```python
from build123d import *

# Parameters (mm, degrees)
F0_R      = 30
F1_DEPTH  = 5
F3_DEPTH  = 95
F4_R      = 25
F5_DEPTH  = 5
F6_R      = 37.5
F6_R_2    = 25
F7_DEPTH  = 10
F8_R      = 25
F9_DEPTH  = 30
F10_R     = 37.5
F11_DEPTH = 10
F12_R     = 25
F13_DEPTH = 5
F15_DEPTH = 95
F16_R     = 30
F17_DEPTH = 5
F18_R     = 20
F19_DEPTH = 30
F20_R     = 20
F21_DEPTH = 30
F22_R     = 10


with BuildPart() as f1:
    # F0 (on Right) → F1 (new body)
    with BuildSketch(Plane.YZ):
        Circle(F0_R)
    extrude(amount=F1_DEPTH)

    # F2 (on face) → F3 (join)
    with BuildSketch(Plane.YZ.offset(5)):
        with BuildLine():
            ThreePointArc((60.0712170477, -35.9367344428), (67.4721616422, -18.6415504541), (70, 0))
            ThreePointArc((70, 0), (37.1422350498, 59.333417022), (-30.5844107288, 62.9650206096))
            Line((-30.5844107288, 62.9650206096), (60.0712170477, -35.9367344428))
        make_face()
        with BuildLine():
            Line((60.0712170477, -35.9367344428), (-30.5844107288, 62.9650206096))
            ThreePointArc((-30.5844107288, 62.9650206096), (-47.2995007919, 51.601911058), (-60.0712170477, 35.9367344428))
            Line((-60.0712170477, 35.9367344428), (30.5844107288, -62.9650206096))
            ThreePointArc((30.5844107288, -62.9650206096), (47.2995007919, -51.601911058), (60.0712170477, -35.9367344428))
        make_face()
        with BuildLine():
            ThreePointArc((-60.0712170477, 35.9367344428), (-47.2995007919, 51.601911058), (-30.5844107288, 62.9650206096))
            Line((-30.5844107288, 62.9650206096), (-39.3131691742, 72.4877557211))
            Line((-39.3131691742, 72.4877557211), (-68.7999754931, 45.4594695543))
            Line((-68.7999754931, 45.4594695543), (-60.0712170477, 35.9367344428))
        make_face()
        with BuildLine():
            Line((68.7999754931, -45.4594695543), (60.0712170477, -35.9367344428))
            ThreePointArc((60.0712170477, -35.9367344428), (47.2995007919, -51.601911058), (30.5844107288, -62.9650206096))
            Line((30.5844107288, -62.9650206096), (39.3131691742, -72.4877557211))
            Line((39.3131691742, -72.4877557211), (68.7999754931, -45.4594695543))
        make_face()
        with BuildLine():
            Line((30.5844107288, -62.9650206096), (-60.0712170477, 35.9367344428))
            ThreePointArc((-60.0712170477, 35.9367344428), (-51.601911058, -47.2995007919), (30.5844107288, -62.9650206096))
        make_face()
    extrude(amount=F3_DEPTH)

    # F4 (on face) → F5 (join)
    with BuildSketch(Plane.YZ.offset(100)):
        Circle(F4_R)
    extrude(amount=F5_DEPTH)

    # F6 (on face) → F7 (join)
    with BuildSketch(Plane.YZ.offset(105)):
        Circle(F6_R)
        Circle(F6_R_2, mode=Mode.SUBTRACT)
        Circle(F6_R_2)
    extrude(amount=F7_DEPTH)

    # F8 (on face) → F9 (join)
    with BuildSketch(Plane.YZ.offset(115)):
        Circle(F8_R)
    extrude(amount=F9_DEPTH)

    # F10 (on face) → F11 (join)
    with BuildSketch(Plane.YZ.offset(145)):
        Circle(F10_R)
    extrude(amount=F11_DEPTH)

    # F12 (on face) → F13 (join)
    with BuildSketch(Plane.YZ.offset(155)):
        Circle(F12_R)
    extrude(amount=F13_DEPTH)

    # F14 (on face) → F15 (join)
    with BuildSketch(Plane.YZ.offset(160)):
        with BuildLine():
            Line((72.4877557211, 39.3131691742), (45.4594695543, 68.7999754931))
            Line((45.4594695543, 68.7999754931), (35.9367344428, 60.0712170477))
            ThreePointArc((35.9367344428, 60.0712170477), (51.601911058, 47.2995007919), (62.9650206096, 30.5844107288))
            Line((62.9650206096, 30.5844107288), (72.4877557211, 39.3131691742))
        make_face()
        with BuildLine():
            ThreePointArc((62.9650206096, 30.5844107288), (51.601911058, 47.2995007919), (35.9367344428, 60.0712170477))
            Line((35.9367344428, 60.0712170477), (-62.9650206096, -30.5844107288))
            ThreePointArc((-62.9650206096, -30.5844107288), (-51.601911058, -47.2995007919), (-35.9367344428, -60.0712170477))
            Line((-35.9367344428, -60.0712170477), (62.9650206096, 30.5844107288))
        make_face()
        with BuildLine():
            Line((-62.9650206096, -30.5844107288), (35.9367344428, 60.0712170477))
            ThreePointArc((35.9367344428, 60.0712170477), (-47.2995007919, 51.601911058), (-62.9650206096, -30.5844107288))
        make_face()
        with BuildLine():
            ThreePointArc((70, 0), (68.2185877993, 15.6915352551), (62.9650206096, 30.5844107288))
            Line((62.9650206096, 30.5844107288), (-35.9367344428, -60.0712170477))
            ThreePointArc((-35.9367344428, -60.0712170477), (34.5284563006, -60.8915897764), (70, 0))
        make_face()
        with BuildLine():
            ThreePointArc((-35.9367344428, -60.0712170477), (-51.601911058, -47.2995007919), (-62.9650206096, -30.5844107288))
            Line((-62.9650206096, -30.5844107288), (-72.4877557211, -39.3131691742))
            Line((-72.4877557211, -39.3131691742), (-45.4594695543, -68.7999754931))
            Line((-45.4594695543, -68.7999754931), (-35.9367344428, -60.0712170477))
        make_face()
    extrude(amount=F15_DEPTH)

    # F16 (on face) → F17 (join)
    with BuildSketch(Plane.YZ.offset(255)):
        Circle(F16_R)
    extrude(amount=F17_DEPTH)

    # F18 (on face) → F19 (join)
    with BuildSketch(Plane(origin=(0, 0, 0), x_dir=(0, -1, 0), z_dir=(-1, 0, 0))):
        Circle(F18_R)
    extrude(amount=F19_DEPTH)

    # F20 (on face) → F21 (join)
    with BuildSketch(Plane.YZ.offset(260)):
        Circle(F20_R)
    extrude(amount=F21_DEPTH)

    # F22
    f22_edges = [f1.edges().sort_by_distance(p)[0] for p in [
        (52.5, -60.071217, 35.936734),
        (207.5, -62.965021, -30.584411),
        (52.5, -30.584411, 62.965021),
        (207.5, 35.936734, 60.071217),
        (207.5, 62.965021, 30.584411),
        (52.5, 60.071217, -35.936734),
        (52.5, 30.584411, -62.965021),
        (207.5, -35.936734, -60.071217),
    ]]
    fillet(f22_edges, radius=F22_R)


solid = f1.part
```
Geometry check sheet. Reference: the model listing, model coordinates, mm. A direction names the side the tool comes from. Give positions to 0.01 mm unless a question says otherwise; leave off trailing zeros. Order: outer loops, then holes, each group sorted by start corner. A loop starts at its lowest first (then second) coordinate and runs counter-clockwise, first axis right, second up. Notation, with made-up numbers: (47.5, 86.5) - (59.5, 86.5) arc R29 ccw to (59.5, 120.5) - close; hole circle Ø6 at (-8, 81.25). An arc over 180 degrees is marked (long way). Write item = value, one per line. Start each with the question number.
1) Section check B-B (x = 61). Enter the section's corners in (y, z), then the cut area to 3 significant figures.
2) Draft check along Y on faces 1 (the cylindrical face through (53.16, -30.25, 65.2)), 2 (the flat face through (155, 24, -8)), 3 (the cylindrical face through (-14.79, 4.336, -19.524)). Enter one of: released by +Y, released by -Y, zero draft, split by the parting line, or undercut.
3) Scan lines: L1, parallel to X at y = -13.5, z = 27; L2, parallel to X at y = -16, z = -65.5; L3, parallel to X at y = 47, z = 54.5. Record each from-to range of solid material in increasing order.
4) Access from +Z, -Z, +X, -X, +Y, -Y to the whole of each face (thin tool, end or side, straight path). Record for faces 4 (the cylindrical face through (2.46, -29.97, 1.32)), 5 (the flat face through (51.835, 53.85, -59.163)), 6 (the flat face through (115, 24, -8)), 7 (the cylindrical face through (257.46, -29.97, 1.32)).
5) Gauge pin test, flat ends, axial feed: pin 1 Ø4 at (x, z) = (14, 53.5) entering from +Y; pin 2 Ø5 at (x, z) = (114.5, 1) entering from +Y; pin 3 Ø12 at (x, z) = (249, -30) entering from -Y. Record the tip position at first contact, or that the pin passes through.
6) Section check A-A (y = -57.5). Enter the section's corners in (x, z), then the cut area to 3 significant figures.
Geometry check:
q1.outline = (-68.8, 45.46) - (-64.86, 41.16) arc R10 cw to (-63.2, 30.1) arc R70 ccw to (24.5, -65.57) arc R10 cw to (35.37, -68.18) - (39.31, -72.49) - (68.8, -45.46) - (64.86, -41.16) arc R10 cw to (63.2, -30.1) arc R70 ccw to (-24.5, 65.57) arc R10 cw to (-35.37, 68.18) - (-39.31, 72.49) - close
q1.area = 16,300 mm2
q2.face_1 = undercut
q2.face_2 = zero draft
q2.face_3 = split by the parting line
q3.L1 = 5 to 100, 105 to 115, 145 to 155, 160 to 255
q3.L2 = 5 to 100, 160 to 255
q3.L3 = 160 to 255
q4.face_4 = -X
q4.face_5 = -Z, +X, -X, +Y
q4.face_6 = none
q4.face_7 = +X
q5.pin_1 = 47.41
q5.pin_2 = 37.5
q5.pin_3 = -68.87
q6.outline = (5, -39.92) - (100, -39.92) - (100, 55.82) - (5, 55.82) - close; (160, -55.66) - (255, -55.66) - (255, 39.92) - (160, 39.92) - close
q6.area = 18,200 mm2
